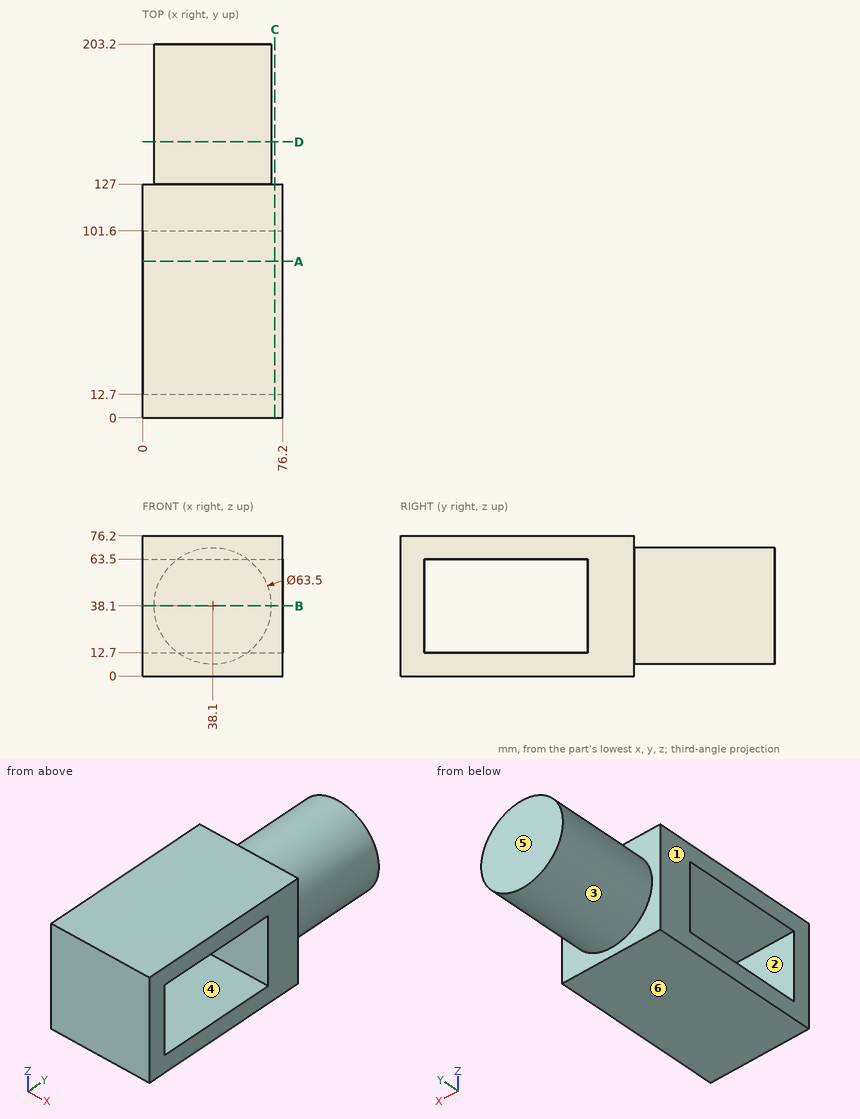
Design review of the part shown in the three views and the two pictorial views. Dimensions are in mm from the part's minimum x, y and z. A direction names the side the tool comes from. Give positions to 0.01 mm unless a question says otherwise; leave off trailing zeros. Write each loop counter-clockwise with the first axis right and the second up, starting at its lowest first coordinate (ties: lowest second). Pieces come first, ordered by that corner, then holes.
(1) Clearance check with flat-ended pins moving along their axes: pin 1 Ø2 at (y, z) = (148, 52.5) entering from -X; pin 2 Ø1 at (x, y) = (24.5, 182) entering from -Z. State where each tip first meets the part, or that it passes through.
Checked values:
pin 1: stops at x = 9.32
pin 2: stops at z = 9.18
(2) Tool access review of the marked faces 1, 2 and 3: name each direction out of +Z, -Z, +X, -X, +Y, -Y from which nothing blocks a thin tool from reaching the whole face with its end or side.
Checked values:
face 1: +Z, -Z, -X, +Y, -Y
face 2: +X, -X
face 3: +Y
(3) Add section C-C (x = 72). Give the boundary of the cut face in (y, z).
Checked values:
outline: (0, 0) - (127, 0) - (127, 76.2) - (0, 76.2) - close; hole (12.7, 12.7) - (101.6, 12.7) - (101.6, 63.5) - (12.7, 63.5) - close
(4) Add section A-A (y = 85). Give the boundary of the cut face in (x, z).
Checked values:
outline: (0, 0) - (76.2, 0) - (76.2, 12.7) - (0, 12.7) - close; (0, 63.5) - (76.2, 63.5) - (76.2, 76.2) - (0, 76.2) - close
(5) Add section D-D (y = 150). Give the boundary of the cut face in (x, z).
Checked values:
outline: circle Ø63.5 at (38.1, 38.1)
(6) Add section B-B (z = 38.1). Give the boundary of the cut face in (x, y).
Checked values:
outline: (0, 0) - (76.2, 0) - (76.2, 12.7) - (0, 12.7) - close; (0, 101.6) - (76.2, 101.6) - (76.2, 127) - (69.85, 127) - (69.85, 203.2) - (6.35, 203.2) - (6.35, 127) - (0, 127) - close
(7) Wall thickness on line 1 along Y through (x, z) = (22, 38); line 2 along Z through (x, y) = (59.5, 61.5); line 3 along Y through (x, z) = (4.5, 30): over which ranges is each line inside the solid? List them lowest first.
Checked values:
line 1: y = 0 to 12.7, 101.6 to 203.2
line 2: z = 0 to 12.7, 63.5 to 76.2
line 3: y = 0 to 12.7, 101.6 to 127
(8) Mouldability with a two-part tool opening along Z and no side actions: class the marked faces 4, 5 and 6 as +Z half, -Z half, draft (parallel to the pull), parting line (faces both ways), or undercut.
Checked values:
face 4: undercut
face 5: draft
face 6: -Z half
